from build123d import *

# Parameters (mm, degrees)
F0_R     = 28.575
F0_R_2   = 25.4
F3_DEPTH = 5.08
F0_R_3   = 31.75
F4_DEPTH = 25.4
F5_R     = 31.75
F5_R_2   = 28.575
F6_DEPTH = 25.4
F7_DEPTH = 5.08


with BuildPart() as f2:
    # F2: sweep along a path in F1
    with BuildLine(Plane.XY) as f2_path:
        Line((0, 0), (0, 19.2369265472))
        ThreePointArc((0, 19.2369265472), (5.8003796226, 48.3974040934), (22.3184632736, 73.1184632736))
        Line((22.3184632736, 73.1184632736), (35.9210244843, 86.7210244843))
    # F0 (on Front) → F2 (sweep)
    with BuildSketch(Plane.XZ):
        Circle(F0_R)
        Circle(F0_R_2, mode=Mode.SUBTRACT)
    sweep(path=f2_path.line)

    # F0 (on Front) → F3 (join)
    with BuildSketch(Plane.XZ):
        Circle(F0_R)
        Circle(F0_R_2, mode=Mode.SUBTRACT)
    extrude(amount=F3_DEPTH)

    # F0 (on Front) → F4 (join)
    with BuildSketch(Plane.XZ):
        Circle(F0_R_3)
        Circle(F0_R, mode=Mode.SUBTRACT)
    extrude(amount=F4_DEPTH)

    # F5 (on face) → F6 (join)
    with BuildSketch(Plane(origin=(61.3210244843, 61.3210244843, 0), x_dir=(-0.7071067812, 0.7071067812, 0), z_dir=(0.7071067812, 0.7071067812, 0))):
        with Locations((35.9210244843, 0)):
            Circle(F5_R)
        with Locations((35.9210244843, 0)):
            Circle(F5_R_2, mode=Mode.SUBTRACT)
    extrude(amount=F6_DEPTH)

    # F7 (add): a face of the model
    f7_faces = [f2.faces().sort_by_distance(p)[0] for p in [
        (35.9210244843, 86.7210244843, -27.7667769491),
    ]]
    extrude(f7_faces, amount=F7_DEPTH)


solid = f2.part
Source: CAD feature listing. Evaluate the final solid. Frame: model axes, mm. A direction names the side the tool comes from. Coordinates: 2 decimals unless noted, no trailing zeros. Loops run counter-clockwise (first coordinate to the right, second up) from the corner with the lowest first, then second, coordinate; pieces in that order, holes last. Notation, with made-up numbers: (4.5, -7) - (41.5, -7) arc R7 cw to (41.5, 5) - close; hole circle Ø11 at (18.5, 66.25). An arc over 180 degrees is marked (long way). Return JSON: item names as keys, results as strings.
Q1. Contact query for flat-ended pins moving along their axis: P1, Ø6, axis at x = 28, y = 62.5, coming from the -Z side; P2, Ø4, axis at y = 43.5, z = 4.5, coming from the +X side; P3, Ø10, axis at x = 46.5, y = 75, coming from the +Z side. Output: stop coordinate, or through.
Results:
{"P1": "z = -27.3", "P2": "x = 36.09", "P3": "z = 29.84"}
Q2. Section B-B, the plane y = -9.5. Return loops of the section in (x, z) (3 decimals), plus the area to 3 significant figures.
Results:
{"outline": "circle Ø63.5 at (0, 0); hole circle Ø57.15 at (0, 0)", "area": "602 mm2"}
Q3. Section D-D, the plane y = 13. Return loops of the section in (x, z) (3 decimals).
Results:
{"outline": "circle Ø57.15 at (0, 0); hole circle Ø50.8 at (0, 0)"}
Q4. Mould query, pull axis Y, two halves, no side actions, for faces 1 (the flat face through (55.98, 66.66, 4.85)), 2 (the cylindrical face through (-5.506, 7.249, -24.796)), 3 (the flat face through (-26, -5.08, -2)). Classes: released by +Y, released by -Y, zero draft, split by the parting line, or undercut.
Results:
{"face 1": "undercut", "face 2": "zero draft", "face 3": "released by -Y"}
Q5. Material intervals for line 1 along Z through (x, y) = (0, -16.75) (3 decimals); line 2 along Z through (x, y) = (0, 1) (3 decimals), sorted ascending.
Results:
{"line 1": "-31.75 to -28.575, 28.575 to 31.75", "line 2": "-28.575 to -25.4, 25.4 to 28.575"}
Q6. Access query for faces 4 (the flat face through (-28.4, -25.4, 4.9)), 5 (the cylindrical face through (-28.547, -15.098, 1.256)), 6 (the cylindrical face through (-28.547, 9.753, -1.256)). Directions: +Z, -Z, +X, -X, +Y, -Y. A direction counts if a zero-diameter tool reaches every point of the face in a straight line with its end or side. Return the directions, or none.
Results:
{"face 4": "+Z, -Z, +X, -X, -Y", "face 5": "-Y", "face 6": "none"}
